from build123d import *

# Parameters (mm, degrees)
CROQUIS1_W                 = 70
CROQUIS1_H                 = 70
SALIENTE_EXTRUIR1_DEPTH    = 20
CROQUIS2_W                 = 45
CROQUIS2_H                 = 45
CORTAR_EXTRUIR1_DEPTH      = 2.5
CORTAR_EXTRUIR2_DEPTH      = 12.5
CORTAR_EXTRUIR2_DEPTH_BACK = 2
CROQUIS3_W                 = 6
CROQUIS3_H                 = 70
CROQUIS4_W                 = 30
CROQUIS4_H                 = 45
CORTAR_EXTRUIR3_DEPTH      = 12
CROQUIS5_R                 = 3
CROQUIS5_R_2               = 1
CORTAR_EXTRUIR4_DEPTH      = 11


with BuildPart() as part:
    # Croquis1 → Saliente-Extruir1 (new body)
    with BuildSketch(Plane(origin=(0, 0, 0), x_dir=(1, 0, 0), z_dir=(0, 1, 0))):
        with Locations((35, 35)):
            Rectangle(CROQUIS1_W, CROQUIS1_H)
    extrude(amount=SALIENTE_EXTRUIR1_DEPTH)

    # Croquis2 → Cortar-Extruir1 (cut)
    with BuildSketch(Plane(origin=(0, 20, 0), x_dir=(1, 0, 0), z_dir=(0, 1, 0))):
        with Locations((35, 35)):
            Rectangle(CROQUIS2_W, CROQUIS2_H)
    extrude(amount=-CORTAR_EXTRUIR1_DEPTH, mode=Mode.SUBTRACT)

    # Croquis3 → Cortar-Extruir2 (cut, two sides: drawn at the far end of the back side and taken through both)
    with BuildSketch(Plane(origin=(0, 17.5, 0), x_dir=(1, 0, 0), z_dir=(0, 1, 0)).offset(-CORTAR_EXTRUIR2_DEPTH_BACK)):
        with Locations((53, 35)):
            Rectangle(CROQUIS3_W, CROQUIS3_H)
        with Locations((17, 35)):
            Rectangle(CROQUIS3_W, CROQUIS3_H)
    extrude(amount=CORTAR_EXTRUIR2_DEPTH + CORTAR_EXTRUIR2_DEPTH_BACK, mode=Mode.SUBTRACT)

    # Croquis4 → Cortar-Extruir3 (cut)
    with BuildSketch(Plane(origin=(0, 17.5, 0), x_dir=(1, 0, 0), z_dir=(0, 1, 0))):
        with Locations((35, 35)):
            Rectangle(CROQUIS4_W, CROQUIS4_H)
    extrude(amount=-CORTAR_EXTRUIR3_DEPTH, mode=Mode.SUBTRACT)

    # Croquis5 → Cortar-Extruir4 (cut)
    with BuildSketch(Plane(origin=(0, 5.5, 0), x_dir=(1, 0, 0), z_dir=(0, 1, 0))):
        with Locations(Location((28, 17.5, 0), (0, 0, 270))):
            Circle(CROQUIS5_R)
        with Locations(Location((42, 17.5, 0), (0, 0, 270))):
            Circle(CROQUIS5_R)
        with Locations(Location((42, 52.5, 0), (0, 0, 90))):
            Circle(CROQUIS5_R)
        with Locations(Location((28, 52.5, 0), (0, 0, 90))):
            Circle(CROQUIS5_R)
        with Locations(Location((35, 35, 0), (0, 0, 270))):
            Circle(CROQUIS5_R_2)
    extrude(amount=-CORTAR_EXTRUIR4_DEPTH, mode=Mode.SUBTRACT)


solid = part.part
Check sheet for the modelled part. Datum: model origin and axes. Units: mm. A direction names the side the tool comes from. Round coordinates to 2 decimals unless told otherwise and drop trailing zeros. Loops run counter-clockwise (first coordinate to the right, second up) from the corner with the lowest first, then second, coordinate; pieces in that order, holes last. Notation, with made-up numbers: (35, 67.5) -> (42, 67.5) arc R21 ccw to (42, 84.5) -> close; hole circle Ø9 at (-10, -15). An arc over 180 degrees is marked (long way). Put each result on its own line as item: value. Start each with the question number.
1. Section check B-B (z = -52.5). Enter the section's corners in (x, y), plus the area to 4 significant figures.
2. Gauge pin test, flat ends, axial feed: pin 1 (5.5 mm diameter, centred on x = 42, z = -17.5, fed in from -Y); pin 2 (6.5 mm diameter, centred on x = 18, z = -48, fed in from +Y); pin 3 (1.2 mm diameter, centred on x = 56.5, z = -26, fed in from +Y). Record the tip position at first contact, or that the pin passes through.
3. Access from +Z, -Z, +X, -X, +Y, -Y to the whole of each face (thin tool, end or side, straight path). Record for faces 5 (the face through (35, 13, -12.5)), 6 (the face through (56, 17, -35)), 7 (the face through (35.84, 2.79, -34.46)).
4. Section check A-A (x = 35). Enter the section's corners in (y, z), plus the area to 4 significant figures.
5. Section check D-D (z = -35). Enter the section's corners in (x, y), plus the area to 4 significant figures.
6. Section check C-C (y = 12.5). Enter the section's corners in (x, z).
7. Scan lines: probe 1 along X at (y, z) = (4.3, -52.5); probe 2 along Z at (x, y) = (40, 17.25); probe 3 along X at (y, z) = (15, -32.5). Record each from-to range of solid material in increasing order.
8. Draft check along Z on faces 1 (the face through (39.97, 2.79, -50.29)), 2 (the face through (17, 15.5, -35)), 3 (the face through (57.5, 19, -35)), 4 (the face through (35, 10, 0)). Enter one of: +Z half, -Z half, draft (parallel to the pull), parting line (faces both ways), or undercut.
Findings:
1. outline: (0, 0) -> (25, 0) -> (25, 5.5) -> (20, 5.5) -> (20, 15.5) -> (14, 15.5) -> (14, 17.5) -> (12.5, 17.5) -> (12.5, 20) -> (0, 20) -> close; (31, 0) -> (39, 0) -> (39, 5.5) -> (31, 5.5) -> close; (45, 0) -> (70, 0) -> (70, 20) -> (57.5, 20) -> (57.5, 17.5) -> (56, 17.5) -> (56, 15.5) -> (50, 15.5) -> (50, 5.5) -> (45, 5.5) -> close
1. area: 837.5 mm^2
2. pin 1: passes through
2. pin 2: stops at y = 15.5
2. pin 3: stops at y = 17.5
3. face 5: +Y
3. face 6: +Z, -Z, +Y
3. face 7: +Y, -Y
4. outline: (0, -70) -> (20, -70) -> (20, -57.5) -> (5.5, -57.5) -> (5.5, -36) -> (0, -36) -> close; (0, -34) -> (5.5, -34) -> (5.5, -12.5) -> (20, -12.5) -> (20, 0) -> (0, 0) -> close
4. area: 736.5 mm^2
5. outline: (0, 0) -> (34, 0) -> (34, 5.5) -> (20, 5.5) -> (20, 15.5) -> (14, 15.5) -> (14, 17.5) -> (12.5, 17.5) -> (12.5, 20) -> (0, 20) -> close; (36, 0) -> (70, 0) -> (70, 20) -> (57.5, 20) -> (57.5, 17.5) -> (56, 17.5) -> (56, 15.5) -> (50, 15.5) -> (50, 5.5) -> (36, 5.5) -> close
5. area: 892.5 mm^2
6. outline: (0, -70) -> (70, -70) -> (70, 0) -> (0, 0) -> close; hole (20, -57.5) -> (50, -57.5) -> (50, -12.5) -> (20, -12.5) -> close
7. probe 1: x = 0 to 25, 31 to 39, 45 to 70
7. probe 2: z = -70 to -57.5, -12.5 to 0
7. probe 3: x = 0 to 20, 50 to 70
8. face 1: undercut
8. face 2: draft
8. face 3: undercut
8. face 4: +Z half
